Read the model definition and answer for the solid it produces. Units are mm, in the model's axes. A direction names the side the tool comes from. Coordinates: 2 decimals unless noted, no trailing zeros. Loops run counter-clockwise (first coordinate to the right, second up) from the corner with the lowest first, then second, coordinate; pieces in that order, holes last. Notation, with made-up numbers: (52, 81) -> (57, 81) arc R9 cw to (57, 86) -> close; hole circle Ø11 at (56, 88.5). An arc over 180 degrees is marked (long way). Answer as a JSON object with one key per item and string values. Group by question number.
Q1. The part is cut by section D-D on y = -9.5. Write down the section's boundary in (x, z), and give its area (3 significant figures).
Q2. The part is cut by section C-C on z = -6. Write down the section's boundary in (x, y).
Q3. For faces 4 (the flat face through (-3, 0, -10)), 5 (the cylindrical face through (6, 0, -5)), determine the directions among +Z, -Z, +X, -X, +Y, -Y from which every point of the face is accessible in a straight line to the end or side of a thin tool.
Q4. Determine the mould class of faces 1 (the cylindrical face through (-29.97, 1.32, 4.19)), 2 (the flat face through (6.2, 0.4, 0)), 3 (the cylindrical face through (0.54, -2.44, -0.88)) for opening direction X: released by +X, released by -X, zero draft, split by the parting line, or undercut.
Q5. The part is cut by section A-A on x = 0. Write down the section's boundary in (y, z).
Q6. Straight lines are drawn through the part: line 1 along Y through (x, z) = (0, -0.5); line 2 along Y through (x, z) = (0, 4); line 3 along Z through (x, y) = (-12, -11). For each, find the intervals that lie inside material, in ascending order. Write a range as [from, to].
Q7. Each of these flat-tipped pins is pushed along its axis until it touches: P1, Ø3, axis at x = -15.5, z = 3.5, coming from the -Y side; P2, Ø6, axis at x = -7.5, y = 22, coming from the -Z side; P3, Ø4, axis at x = 0, y = 0, coming from the -Z side; P4, Ø8, axis at x = 12.5, z = 3, coming from the +Y side. Where does it stop, or does it pass through?
from build123d import *

# Parameters (mm, degrees)
SKETCH1_R           = 30
BOSS_EXTRUDE1_DEPTH = 8.5
SKETCH2_R           = 6
SKETCH2_R_2         = 2.5
BOSS_EXTRUDE2_DEPTH = 10
SKETCH3_R           = 2.5
CUT_EXTRUDE1_DEPTH  = 19.5


with BuildPart() as part:
    # Sketch1 → Boss-Extrude1 (new body)
    with BuildSketch(Plane.XY):
        Circle(SKETCH1_R)
    extrude(amount=BOSS_EXTRUDE1_DEPTH)

    # Sketch2 → Boss-Extrude2 (add)
    with BuildSketch(Plane(origin=(0, 0, 0), x_dir=(-1, 0, 0), z_dir=(0, 0, -1))):
        Circle(SKETCH2_R)
        Circle(SKETCH2_R_2, mode=Mode.SUBTRACT)
    extrude(amount=BOSS_EXTRUDE2_DEPTH)

    # Sketch3 → Cut-Extrude1 (cut, through all)
    with BuildSketch(Plane(origin=(0, 0, -10), x_dir=(-1, 0, 0), z_dir=(0, 0, -1))):
        Circle(SKETCH3_R)
    extrude(amount=-CUT_EXTRUDE1_DEPTH, mode=Mode.SUBTRACT)


solid = part.part
Final values:
{
 "1": {"outline": "(-28.46, 0) -> (28.46, 0) -> (28.46, 8.5) -> (-28.46, 8.5) -> close", "area": "484 mm2"},
 "2": {"outline": "circle Ø12 at (0, 0); hole circle Ø5 at (0, 0)"},
 "3": {"face 4": "-Z, +X, -X, +Y, -Y", "face 5": "-Z"},
 "4": {"face 1": "split by the parting line", "face 2": "zero draft", "face 3": "undercut"},
 "5": {"outline": "(-30, 0) -> (-6, 0) -> (-6, -10) -> (-2.5, -10) -> (-2.5, 8.5) -> (-30, 8.5) -> close; (2.5, -10) -> (6, -10) -> (6, 0) -> (30, 0) -> (30, 8.5) -> (2.5, 8.5) -> close"},
 "6": {"line 1": "y = [-6, -2.5], [2.5, 6]", "line 2": "y = [-30, -2.5], [2.5, 30]", "line 3": "z = [0, 8.5]"},
 "7": {"P1": "stops at y = -26.53", "P2": "stops at z = 0", "P3": "passes through", "P4": "stops at y = 28.77"}
}
